Part model, mm, in its own coordinate system. Face numbers are marked on the shaded views. Coordinates: 2 decimals unless noted, no trailing zeros. Loops run counter-clockwise (first coordinate to the right, second up) from the corner with the lowest first, then second, coordinate; pieces in that order, holes last. Notation, with made-up numbers: M 41,72 L 45,72 A20 cw 45,85 Z; hole C 89.25,56 d7. An arc over 180 degrees is marked long. Use a Markdown table: item, result. Add a question column.
1) Band-saw the part on B-B (x = 0). List the corners of the cut face in (y, z).
2) Band-saw the part on C-C (z = -25.4). List the corners of the cut face in (x, y), plus the area to 3 significant figures.
3) Band-saw the part on D-D (z = -10.5). List the corners of the cut face in (x, y), plus the area to 3 significant figures.
4) Pull direction Y, two halves, no side cores. Call the marked faces 1, 2 and 3: released by +Y, released by -Y, zero draft, split by the parting line, or undercut.
5) Pin check, flat tips, straight feed: pin 1 Ø8 at (x, z) = (14.5, -22.5) entering from +Y; pin 2 Ø3 at (x, z) = (13.5, -26.5) entering from +Y. Stop position of each tip, or through.
6) Wall check: probe 1 along X at (y, z) = (3.65, -25.4); probe 2 along X at (y, z) = (2.54, 33.8); probe 3 along Z at (x, y) = (11, 12). Give the ranges that are in metal, low to high. Write a range as from..to.
7) Band-saw the part on A-A (y = 8.75). List the corners of the cut face in (x, z), plus the area to 3 significant figures.
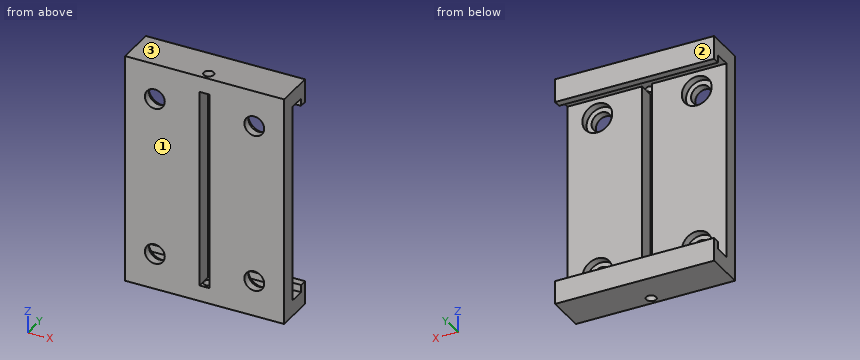
from build123d import *

# Parameters (mm, degrees)
SKETCH1_W           = 50.8
SKETCH1_H           = 73.66
BOSS_EXTRUDE1_DEPTH = 25.4
SKETCH4_W           = 63.5
SKETCH4_H           = 5.08
SKETCH4_W_2         = 58.7375
SKETCH4_H_2         = 2.38125
CUT_EXTRUDE3_DEPTH  = 51.8
SKETCH5_W           = 73.66
SKETCH5_H           = 12.85875
CUT_EXTRUDE4_DEPTH  = 51.8
SKETCH6_W           = 3.175
SKETCH6_H           = 63.5
CUT_EXTRUDE5_DEPTH  = 6.08
SKETCH7_R           = 3.175
CUT_EXTRUDE6_DEPTH  = 6.08
SKETCH8_R           = 4.7625
CUT_EXTRUDE7_DEPTH  = 2.54
SKETCH9_R           = 1.5875
CUT_EXTRUDE8_DEPTH  = 68.58


with BuildPart() as part:
    # Sketch1 → Boss-Extrude1 (new body)
    with BuildSketch(Plane(origin=(0, 0, 0), x_dir=(1, 0, 0), z_dir=(0, 1, 0))):
        Rectangle(SKETCH1_W, SKETCH1_H)
    extrude(amount=BOSS_EXTRUDE1_DEPTH)

    # Sketch4 → Cut-Extrude3 (cut, through all)
    with BuildSketch(Plane(origin=(25.4, 0, 0), x_dir=(0, 0, -1), z_dir=(1, 0, 0))):
        with Locations((0, 7.62)):
            Rectangle(SKETCH4_W, SKETCH4_H)
        with Locations((0, 11.350625)):
            Rectangle(SKETCH4_W_2, SKETCH4_H_2)
    extrude(amount=-CUT_EXTRUDE3_DEPTH, mode=Mode.SUBTRACT)

    # Sketch5 → Cut-Extrude4 (cut, through all)
    with BuildSketch(Plane(origin=(25.4, 0, 0), x_dir=(0, 0, -1), z_dir=(1, 0, 0))):
        with Locations((0, 18.970625)):
            Rectangle(SKETCH5_W, SKETCH5_H)
    extrude(amount=-CUT_EXTRUDE4_DEPTH, mode=Mode.SUBTRACT)

    # Sketch6 → Cut-Extrude5 (cut, through all)
    with BuildSketch(Plane(origin=(0, 5.08, 0), x_dir=(1, 0, 0), z_dir=(0, 1, 0))):
        Rectangle(SKETCH6_W, SKETCH6_H)
    extrude(amount=-CUT_EXTRUDE5_DEPTH, mode=Mode.SUBTRACT)

    # Sketch7 → Cut-Extrude6 (cut, through all)
    with BuildSketch(Plane(origin=(0, 5.08, 0), x_dir=(1, 0, 0), z_dir=(0, 1, 0))):
        with Locations((15.875, 25.4)):
            Circle(SKETCH7_R)
        with Locations((-15.875, 25.4)):
            Circle(SKETCH7_R)
        with Locations((-15.875, -25.4)):
            Circle(SKETCH7_R)
        with Locations((15.875, -25.4)):
            Circle(SKETCH7_R)
    extrude(amount=-CUT_EXTRUDE6_DEPTH, mode=Mode.SUBTRACT)

    # Sketch8 → Cut-Extrude7 (cut)
    with BuildSketch(Plane(origin=(0, 5.08, 0), x_dir=(1, 0, 0), z_dir=(0, 1, 0))):
        with Locations((-15.875, 25.4)):
            Circle(SKETCH8_R)
        with Locations((-15.875, -25.4)):
            Circle(SKETCH8_R)
        with Locations((15.875, -25.4)):
            Circle(SKETCH8_R)
        with Locations((15.875, 25.4)):
            Circle(SKETCH8_R)
    extrude(amount=-CUT_EXTRUDE7_DEPTH, mode=Mode.SUBTRACT)

    # Sketch9 → Cut-Extrude8 (cut)
    with BuildSketch(Plane.XY.offset(36.83)):
        with Locations((0, 2.54)):
            Circle(SKETCH9_R)
    cut_extrude8 = extrude(amount=-CUT_EXTRUDE8_DEPTH, mode=Mode.SUBTRACT)

    # Mirror1: Cut-Extrude8 across plane
    add(cut_extrude8.mirror(Plane.XY), mode=Mode.SUBTRACT)


solid = part.part
Entries:
| question | item | result |
|---|---|---|
| 1 | outline | M 0,-36.83 L 0.95,-36.83 L 0.95,-31.75 L 0,-31.75 Z; M 0,31.75 L 0.95,31.75 L 0.95,36.83 L 0,36.83 Z; M 4.13,-36.83 L 12.54,-36.83 L 12.54,-29.37 L 10.16,-29.37 L 10.16,-31.75 L 4.13,-31.75 Z; M 4.13,31.75 L 10.16,31.75 L 10.16,29.37 L 12.54,29.37 L 12.54,36.83 L 4.13,36.83 Z |
| 2 | outline | M -25.4,0 L -19.05,0 L -19.05,2.54 L -20.64,2.54 L -20.64,5.08 L -25.4,5.08 Z; M -12.7,0 L -1.59,0 L -1.59,5.08 L -11.11,5.08 L -11.11,2.54 L -12.7,2.54 Z; M 1.59,0 L 12.7,0 L 12.7,2.54 L 11.11,2.54 L 11.11,5.08 L 1.59,5.08 Z; M 19.05,0 L 25.4,0 L 25.4,5.08 L 20.64,5.08 L 20.64,2.54 L 19.05,2.54 Z |
| 2 | area | 161 mm2 |
| 3 | outline | M -25.4,0 L -1.59,0 L -1.59,5.08 L -25.4,5.08 Z; M 1.59,0 L 25.4,0 L 25.4,5.08 L 1.59,5.08 Z |
| 3 | area | 242 mm2 |
| 4 | face 1 | released by -Y |
| 4 | face 2 | released by +Y |
| 4 | face 3 | zero draft |
| 5 | pin 1 | y = 5.08 |
| 5 | pin 2 | y = 2.54 |
| 6 | probe 1 | -25.4..-20.64, -11.11..-1.59, 1.59..11.11, 20.64..25.4 |
| 6 | probe 2 | -25.4..-1.59, 1.59..25.4 |
| 6 | probe 3 | -36.83..-29.37, 29.37..36.83 |
| 7 | outline | M -25.4,-36.83 L 25.4,-36.83 L 25.4,-31.75 L -25.4,-31.75 Z; M -25.4,31.75 L 25.4,31.75 L 25.4,36.83 L -25.4,36.83 Z |
| 7 | area | 516 mm2 |
